Geometry check sheet. Reference: the model listing, model coordinates, mm. Round coordinates to 2 decimals unless told otherwise and drop trailing zeros. Loops run counter-clockwise (first coordinate to the right, second up) from the corner with the lowest first, then second, coordinate; pieces in that order, holes last. Notation, with made-up numbers: (0.5, 49.5) -> (55.5, 49.5) arc R8 cw to (55.5, 56.5) -> close; hole circle Ø5 at (89.25, 26.5). An arc over 180 degrees is marked (long way). Use a Markdown table: item, result. Add a question column.
Q1. Sectioned sample at B-B, the plane x = 8.5. Enter the section's corners in (y, z).
Q2. Gauge pin test, flat ends, axial feed: P1, Ø4, axis at x = -5.5, y = 4.5, coming from the +Z side; P2, Ø1, axis at x = -5, y = 19.5, coming from the +Z side; P3, Ø5, axis at x = 13, y = 9, coming from the -Z side. Record the tip position at first contact, or that the pin passes through.
Q3. Sectioned sample at D-D, the plane y = -6. Enter the section's corners in (x, z).
Q4. Sectioned sample at C-C, the plane x = 4.5. Enter the section's corners in (y, z).
Q5. Release check for a two-part mould opening along Y. For faces 1 (the face through (-1, -0.881, 3)), 2 (the face through (2, 23.498, 4)) record: released by +Y, released by -Y, zero draft, split by the parting line, or undercut.
Q6. Sectioned sample at A-A, the plane y = 5. Enter the section's corners in (x, z).
Q7. Material ranges on L1, parallel to X at y = -1, z = 1.5; L2, parallel to Y at x = -0.5, z = 4.25; L3, parallel to X at y = -10.5, z = 3.5, recorded low to high.
```python
from build123d import *

# Parameters (mm, degrees)
F0_W     = 38.1
F0_H     = 38.1
F1_DEPTH = 0.79375
F2_W     = 38.1
F2_H     = 38.1
F2_W_2   = 34.8996
F2_H_2   = 34.8996
F3_DEPTH = 6.35
F4_W     = 1.27
F4_H     = 17.6995960579
F4_H_2   = 29.188188513
F4_W_2   = 11.795372231
F4_H_3   = 1.27
F4_H_4   = 11.3495960579
F4_H_5   = 5.7700039421
F6_DEPTH = 4.445
F5_R     = 1.27
F7_DEPTH = 0.396875


# Not quite as in the source:
# - a feature names something its author has since deleted; it is built from what else it names


with BuildPart() as f1:
    # F0 (on Top) → F1 (new body)
    with BuildSketch(Plane.XY):
        with Locations((2.218876034, 4.4484467313)):
            Rectangle(F0_W, F0_H)
    extrude(amount=F1_DEPTH)

    # F2 (on face) → F3 (join)
    with BuildSketch(Plane.XY.offset(0.79375)):
        with Locations((2.218876034, 4.4484467313)):
            Rectangle(F2_W, F2_H)
        with Locations((2.218876034, 4.4484467313)):
            Rectangle(F2_W_2, F2_H_2, mode=Mode.SUBTRACT)
    extrude(amount=F3_DEPTH)

    # F4 (on face) → F6 (join)
    with BuildSketch(Plane.XY.offset(0.79375)):
        with Locations((-3.165923966, 13.0484487024)):
            Rectangle(F4_W, F4_H)
        with Locations((-9.515923966, 1.5927409878)):
            Rectangle(F4_W, F4_H_2)
        Polygon((-3.800923966, -2.1513493266), (19.668676034, -2.1513493266), (19.668676034, -0.8813493266), (3.819076034, -0.8813493266), (3.819076034, 5.701588226), (2.549076034, 5.701588226), (2.549076034, -0.8813493266), (-3.800923966, -0.8813493266), align=None)
        Polygon((-3.800923966, -8.5013493266), (-3.800923966, -13.0013532687), (-2.530923966, -13.0013532687), (-2.530923966, -8.5013493266), (5.089076034, -8.5013493266), (5.089076034, -7.2313493266), (3.819076034, -7.2313493266), (-3.800923966, -7.2313493266), align=None)
        Polygon((8.0383015836, 21.8982467313), (6.7683015836, 21.8982467313), (6.7683015836, 12.051588226), (2.549076034, 12.051588226), (2.549076034, 10.781588226), (8.0383015836, 10.781588226), align=None)
        with Locations((13.7709899185, 4.8336506734)):
            Rectangle(F4_W_2, F4_H_3)
        with Locations((13.7533015836, 16.2234487024)):
            Rectangle(F4_W, F4_H_4)
        with Locations((13.953676034, -10.1163512976)):
            Rectangle(F4_W, F4_H_5)
    extrude(amount=F6_DEPTH)

    # F5 (on face) → F7 (cut)
    with BuildSketch(Plane.XY.offset(0.79375)):
        with Locations((17.0904958928, -8.8772866875)):
            Circle(F5_R)
        with Locations((-12.6393535174, -8.3864945918)):
            Circle(F5_R)
    extrude(amount=-F7_DEPTH, mode=Mode.SUBTRACT)


solid = f1.part
```
Values:
| question | item | result |
|---|---|---|
| 1 | outline | (-14.6, 0) -> (23.5, 0) -> (23.5, 7.14) -> (21.9, 7.14) -> (21.9, 0.79) -> (5.47, 0.79) -> (5.47, 5.24) -> (4.2, 5.24) -> (4.2, 0.79) -> (-0.88, 0.79) -> (-0.88, 5.24) -> (-2.15, 5.24) -> (-2.15, 0.79) -> (-13, 0.79) -> (-13, 7.14) -> (-14.6, 7.14) -> close |
| 2 | P1 | z = 5.24 |
| 2 | P2 | z = 0.79 |
| 2 | P3 | z = 0 |
| 3 | outline | (-16.83, 0) -> (21.27, 0) -> (21.27, 7.14) -> (19.67, 7.14) -> (19.67, 0.79) -> (-8.88, 0.79) -> (-8.88, 5.24) -> (-10.15, 5.24) -> (-10.15, 0.79) -> (-15.23, 0.79) -> (-15.23, 7.14) -> (-16.83, 7.14) -> close |
| 4 | outline | (-14.6, 0) -> (23.5, 0) -> (23.5, 7.14) -> (21.9, 7.14) -> (21.9, 0.79) -> (12.05, 0.79) -> (12.05, 5.24) -> (10.78, 5.24) -> (10.78, 0.79) -> (-0.88, 0.79) -> (-0.88, 5.24) -> (-2.15, 5.24) -> (-2.15, 0.79) -> (-7.23, 0.79) -> (-7.23, 5.24) -> (-8.5, 5.24) -> (-8.5, 0.79) -> (-13, 0.79) -> (-13, 7.14) -> (-14.6, 7.14) -> close |
| 5 | face 1 | undercut |
| 5 | face 2 | released by +Y |
| 6 | outline | (-16.83, 0) -> (21.27, 0) -> (21.27, 7.14) -> (19.67, 7.14) -> (19.67, 5.24) -> (7.87, 5.24) -> (7.87, 0.79) -> (3.82, 0.79) -> (3.82, 5.24) -> (2.55, 5.24) -> (2.55, 0.79) -> (-2.53, 0.79) -> (-2.53, 5.24) -> (-3.8, 5.24) -> (-3.8, 0.79) -> (-8.88, 0.79) -> (-8.88, 5.24) -> (-10.15, 5.24) -> (-10.15, 0.79) -> (-15.23, 0.79) -> (-15.23, 7.14) -> (-16.83, 7.14) -> close |
| 7 | L1 | -16.83 to -15.23, -10.15 to -8.88, -3.8 to 21.27 |
| 7 | L2 | -14.6 to -13, -8.5 to -7.23, -2.15 to -0.88, 21.9 to 23.5 |
| 7 | L3 | -16.83 to -15.23, -10.15 to -8.88, -3.8 to -2.53, 13.32 to 14.59, 19.67 to 21.27 |
